Design review of the part built by this model. Coordinates are the model's own, in mm. Give positions to 0.01 mm unless a question says otherwise; leave off trailing zeros. Write each loop counter-clockwise with the first axis right and the second up, starting at its lowest first coordinate (ties: lowest second). Pieces come first, ordered by that corner, then holes.
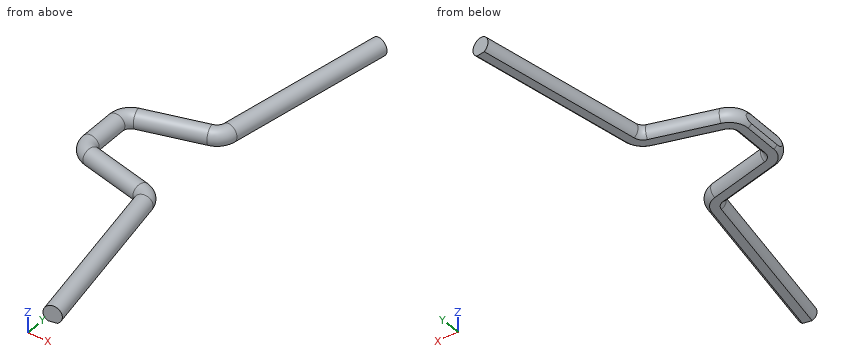
```python
from build123d import *

# Parameters (mm, degrees)
SKETCH_2_R               = 0.75
CUT_EXTRUDE_1_DEPTH      = 23.321950206
CUT_EXTRUDE_1_DEPTH_BACK = 23.321950206
SKETCH_3_W               = 12
SKETCH_3_H               = 0.1
CUT_EXTRUDE_2_DEPTH      = 23.321950206
CUT_EXTRUDE_2_DEPTH_BACK = 23.321950206
SKETCH_4_W               = 0.1
SKETCH_4_H               = 1.5


with BuildPart() as part:
    # По траектории1: sweep along a path in Эскиз1
    with BuildLine(Plane.XY) as sweep_1_path:
        Line((9.683583031, 19.595), (7.138282612, 5.159884012))
        ThreePointArc((7.138282612, 5.159884012), (6.828869592, 4.532456475), (6.230796727, 4.169536951))
        Line((6.230796727, 4.169536951), (0.926476194, 2.748248548))
        ThreePointArc((0.926476194, 2.748248548), (0.258308325, 2.301793051), (0, 1.540841265))
        Line((0, 1.540841265), (0, -1.540841265))
        ThreePointArc((0, -1.540841265), (0.258308325, -2.301793051), (0.926476194, -2.748248548))
        Line((0.926476194, -2.748248548), (6.230796727, -4.169536951))
        ThreePointArc((6.230796727, -4.169536951), (6.828869592, -4.532456475), (7.138282612, -5.159884012))
        Line((7.138282612, -5.159884012), (9.683583031, -19.595))
    # Эскиз2 → По траектории1 (sweep)
    with BuildSketch(Plane(origin=(0, 0, 0), x_dir=(1, 0, 0), z_dir=(0, 1, 0))):
        Circle(SKETCH_2_R)
    sweep(path=sweep_1_path.line)

    # Эскиз3 → Вырез-Вытянуть1 (cut, two sides: drawn at the far end of the back side and taken through both)
    with BuildSketch(Plane(origin=(0, 0, 0), x_dir=(1, 0, 0), z_dir=(0, 1, 0)).offset(-CUT_EXTRUDE_1_DEPTH_BACK)):
        with Locations((5, 0.7)):
            Rectangle(SKETCH_3_W, SKETCH_3_H)
    extrude(amount=CUT_EXTRUDE_1_DEPTH + CUT_EXTRUDE_1_DEPTH_BACK, mode=Mode.SUBTRACT)

    # Эскиз4 → Вырез-Вытянуть2 (cut, two sides: drawn at the far end of the back side and taken through both)
    with BuildSketch(Plane(origin=(0, 0, 0), x_dir=(1, 0, 0), z_dir=(0, 1, 0)).offset(-CUT_EXTRUDE_2_DEPTH_BACK)):
        with Locations((-0.7, 0)):
            Rectangle(SKETCH_4_W, SKETCH_4_H)
    extrude(amount=CUT_EXTRUDE_2_DEPTH + CUT_EXTRUDE_2_DEPTH_BACK, mode=Mode.SUBTRACT)


solid = part.part
```
(1) Clearance check with a flat-ended pin moving along its axis: P1, Ø1.5, axis at x = 4.5, y = -9.5, coming from the +Z side. State where the tip first meets the part, or that it passes through.
Resolved:
P1: passes through
(2) Consider section B-B, the plane y = 1. Give the boundary of the cut face in (x, z).
Resolved:
outline: (-0.65, -0.37) arc R0.75 ccw to (-0.37, -0.65) - (0.37, -0.65) arc R0.75 ccw (long way) to (-0.65, 0.37) - close
(3) To check wall thickness, follow L1, parallel to Y at x = 2, z = -0.15; L2, parallel to Y at x = 6.25, z = -0.25; L3, parallel to X at y = 0.5, z = 0.1. State the ranges of each line that lie inside material, in increasing order.
Resolved:
L1: y = -3.8 to -2.28, 2.28 to 3.8
L2: y = -4.96 to -3.44, 3.44 to 4.96
L3: x = -0.65 to 0.74
(4) Consider section A-A, the plane z = 0.05. Give the boundary of the cut face in (x, y), then the cut area to 3 significant figures.
Resolved:
outline: (-0.65, -2.16) arc R2 ccw to (0.73, -3.47) - (6.04, -4.89) arc R0.5 cw to (6.4, -5.29) - (8.95, -19.72) - (10.42, -19.47) - (7.88, -5.03) arc R2 ccw to (6.42, -3.45) - (1.12, -2.03) arc R0.5 cw to (0.75, -1.54) - (0.75, 1.54) arc R0.5 cw to (1.12, 2.03) - (6.42, 3.45) arc R2 ccw to (7.88, 5.03) - (10.42, 19.47) - (8.95, 19.72) - (6.4, 5.29) arc R0.5 cw to (6.04, 4.89) - (0.73, 3.47) arc R2 ccw to (-0.65, 2.16) - close
area: 73.7 mm2
